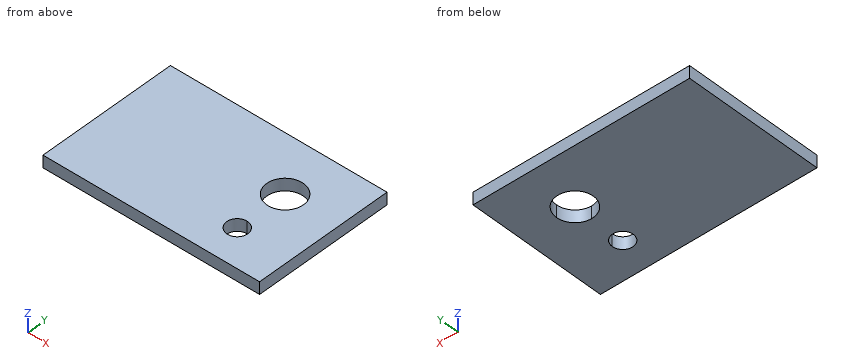
```python
from build123d import *

# Parameters (mm, degrees)
F0_W     = 124
F0_H     = 80
F1_DEPTH = 7
F5_DEPTH = 25


with BuildPart() as f1:
    # F0 (on Top) → F1 (new body)
    with BuildSketch(Plane.XY):
        with Locations((-62, 40)):
            Rectangle(F0_W, F0_H)
    extrude(amount=-F1_DEPTH)


with BuildPart() as f2_1:
    # F2: copy of F1
    add(f1.part)

    # F4 (on face) → F5 (cut)
    with BuildSketch(Plane.XY):
        with BuildLine():
            ThreePointArc((-20.5, 50), (-38.424621, 57.424621), (-31, 39.5))
            ThreePointArc((-31, 39.5), (-23.575379, 42.575379), (-20.5, 50))
        make_face()
        with BuildLine():
            ThreePointArc((-25, 20), (-26.757359, 24.242641), (-31, 26))
            ThreePointArc((-31, 26), (-35.242641, 15.757359), (-25, 20))
        make_face()
    extrude(amount=-F5_DEPTH, mode=Mode.SUBTRACT)


solid = f2_1.part
```
Here's how the part is built. I have some questions about the finished solid (model axes, mm). Give positions to 0.01 mm unless a question says otherwise; leave off trailing zeros. Loops run counter-clockwise (first coordinate to the right, second up) from the corner with the lowest first, then second, coordinate; pieces in that order, holes last. Notation, with made-up numbers: M 87,-34.75 L 122,-34.75 A16 cw 122,-26.75 Z; hole C -14.75,64.5 d8. An arc over 180 degrees is marked long. Use one line per item in the form item = value. Start each with the question number.
Q1. I need wall thicknesses on line 1 along Y through (x, z) = (-30.5, -5.25); line 2 along X through (y, z) = (20, -4.25); line 3 along X through (y, z) = (50, -1.75). Which ranges of each line are inside material? Lowest first, please.
Q2. If we section it at A-A (x = -35.5): Write out the boundary of the cut face in (y, z).
Q3. Will this pin go through, and if not, where does the flat tip stop? pin 1 Ø1.5 at (x, z) = (-20, -4) entering from -Y.
Q4. If we section it at C-C (y = 23.5): Write out the boundary of the cut face in (x, z).
Q5. If we section it at B-B (z = -3): Write out the boundary of the cut face in (x, y).
Taken from the geometry:
q1.line_1 = 0 to 14.02, 25.98 to 39.51, 60.49 to 80
q1.line_2 = -124 to -37, -25 to 0
q1.line_3 = -124 to -41.5, -20.5 to 0
q2.outline = M 0,-7 L 16.03,-7 L 16.03,0 L 0,0 Z; M 23.97,-7 L 40.51,-7 L 40.51,0 L 23.97,0 Z; M 59.49,-7 L 80,-7 L 80,0 L 59.49,0 Z
q3.pin_1 = 0
q4.outline = M -124,-7 L -35.87,-7 L -35.87,0 L -124,0 Z; M -26.13,-7 L 0,-7 L 0,0 L -26.13,0 Z
q5.outline = M -124,0 L 0,0 L 0,80 L -124,80 Z; hole C -31,50 d21; hole M -31,26 A6 ccw long -25,20 A6 ccw Z
